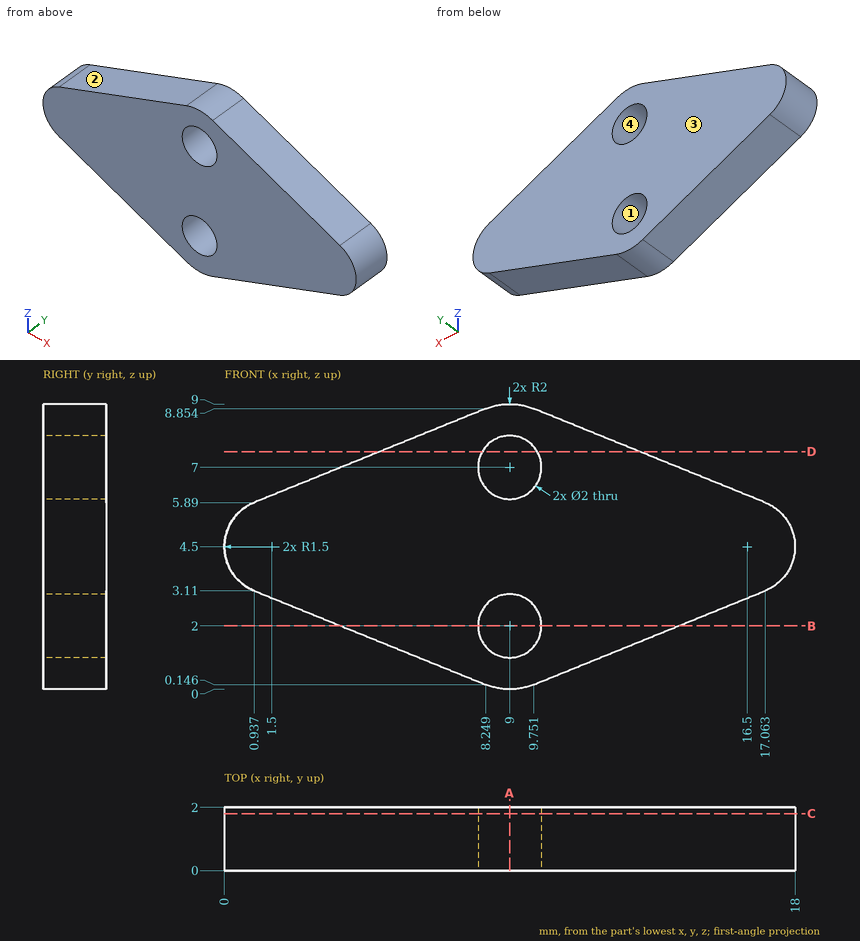
Geometry: see drawing. Coordinates: mm, zero at the bounding-box minimum. Give positions to 0.01 mm unless a question says otherwise; leave off trailing zeros. Loops run counter-clockwise (first coordinate to the right, second up) from the corner with the lowest first, then second, coordinate; pieces in that order, holes last. Notation, with made-up numbers: (-31.75, 11.25) - (-17.75, 11.25) arc R19 ccw to (-17.75, 45.25) - close; hole circle Ø8 at (-21, 5). An arc over 180 degrees is marked (long way). Use CSV: the item, a comma, the result in double quotes.
1) Cut plane A-A (x = 9). Output: boundary loops of the cut face in (y, z), and give its area (3 significant figures).
Worked out:
outline,"(0, 0) - (2, 0) - (2, 1) - (0, 1) - close; (0, 3) - (2, 3) - (2, 6) - (0, 6) - close; (0, 8) - (2, 8) - (2, 9) - (0, 9) - close"
area,"10.0 mm^2"
2) Cut plane D-D (z = 7.5). Output: boundary loops of the cut face in (x, y), and give its area (3 significant figures).
Worked out:
outline,"(4.91, 0) - (8.13, 0) - (8.13, 2) - (4.91, 2) - close; (9.87, 0) - (13.09, 0) - (13.09, 2) - (9.87, 2) - close"
area,"12.9 mm^2"
3) Cut plane C-C (y = 1.8). Output: boundary loops of the cut face in (x, z).
Worked out:
outline,"(0.94, 3.11) - (8.25, 0.15) arc R2 ccw to (9.75, 0.15) - (17.06, 3.11) arc R1.5 ccw to (17.06, 5.89) - (9.75, 8.85) arc R2 ccw to (8.25, 8.85) - (0.94, 5.89) arc R1.5 ccw to start; hole circle Ø2 at (9, 2); hole circle Ø2 at (9, 7)"
4) Mould query, pull axis Z, two halves, no side actions, for the marked faces 1, 2, 3 and 4. Classes: +Z half, -Z half, draft (parallel to the pull), parting line (faces both ways), or undercut.
Worked out:
face 1,"undercut"
face 2,"+Z half"
face 3,"draft"
face 4,"undercut"
5) Cut plane B-B (z = 2). Output: boundary loops of the cut face in (x, y) (1 decimal), and give its area (3 significant figures).
Worked out:
outline,"(3.7, 0) - (8, 0) - (8, 2) - (3.7, 2) - close; (10, 0) - (14.3, 0) - (14.3, 2) - (10, 2) - close"
area,"17.3 mm^2"
6) Pin query (flat end, axial travel): P1, Ø1, axis at y = 1, z = 6.5, coming from the -X side (1 decimal); P2, Ø1.6, axis at x = 9, z = 7, coming from the -Y side; P3, Ø1, axis at y = 0.5, z = 7, coming from the -X side. Return the tip coordinate at first contact, or that it passes through.
Worked out:
P1,"stops at x = 1.2"
P2,"passes through"
P3,"stops at x = 2.44"
7) Line query: line 1 (X direction, y = 0.5, z = 7) (1 decimal); line 2 (X direction, y = 1.9, z = 2.25) (1 decimal); line 3 (X direction, y = 0.2, z = 3.25). Output: solid intervals per line, ascending.
Worked out:
line 1,"x = 3.7 to 8, 10 to 14.3"
line 2,"x = 3.1 to 8, 10 to 14.9"
line 3,"x = 0.67 to 17.33"
